Here's how the part is built. I have some questions about the finished solid (model axes, mm). Face numbers are marked on the shaded views. A direction names the side the tool comes from. Coordinates: 2 decimals unless noted, no trailing zeros. Order: outer loops, then holes, each group sorted by start corner. A loop starts at its lowest first (then second) coordinate and runs counter-clockwise, first axis right, second up. Notation, with made-up numbers: (-3, -23.75) - (3, -23.75) arc R27 cw to (3, 14.25) - close; hole circle Ø5 at (45, 4.25). An arc over 180 degrees is marked (long way). Answer as CSV lines item,"result". Start each with the question number.
Q1. For pin 1 Ø0.8 at (x, y) = (-6.5, -16) entering from +Z; pin 2 Ø1.5 at (x, y) = (4.5, -14.5) entering from +Z; pin 3 Ø5 at (x, y) = (0.5, 8) entering from -Z, each with a flat end and sliding along its axis, tell me the tip position at first contact or that it passes through.
Q2. Suppose I cut it at B-B (y = 14). Please give me the cut outline in (x, z), then the cut area to 3 significant figures.
Q3. Suppose I cut it at A-A (x = -6). Please give me the cut outline in (y, z), then the cut area to 3 significant figures.
Q4. For the marked faces 1, 2, 3, 4 and 5, which set-ups out of +Z, -Z, +X, -X, +Y, -Y let a thin tool reach every point of the face, with its end or its side?
Q5. Suppose I cut it at C-C (z = 0). Please give me the cut outline in (x, y), then the cut area to 3 significant figures.
Q6. I need wall thicknesses on line 1 (Y direction, x = -3.25, z = 10); line 2 (Y direction, x = -5.25, z = 3); line 3 (Z direction, x = -3.5, y = 11). Which ranges of each line are inside material? Lowest first, please.
Q7. Suppose I cut it at D-D (z = 9.5). Please give me the cut outline in (x, y), then the cut area to 3 significant figures.
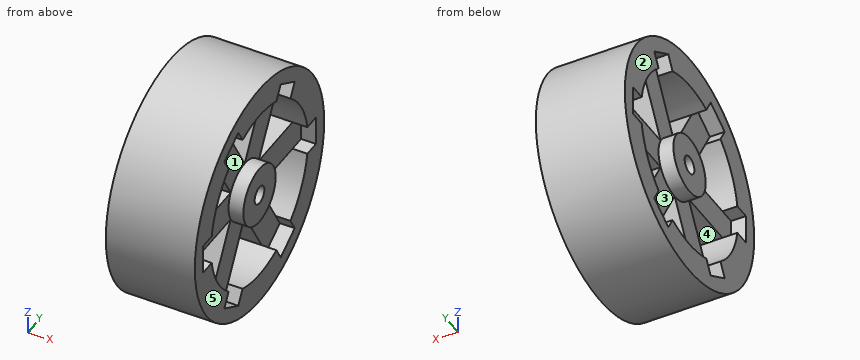
Autodesk Inventor part; units mm, degrees
ref_plane "YZ Plane" through (0, 0, 0) normal (1, 0, 0) x (0, 1, 0)
ref_plane "XZ Plane" through (0, 0, 0) normal (0, 1, 0) x (-1, 0, 0)
ref_plane "XY Plane" through (0, 0, 0) normal (0, 0, 1) x (1, 0, 0)
sketch "Sketch1" plane through (0, 0, 0) normal (1, 0, 0) x (0, 1, 0)
  circle A0 centre (0, 0) radius 20
  circle A1 centre (0, 0) radius 15
  circle A2 centre (0, 0) radius 5
  line L0 (20, 0) -> (9.9317, 0) construction
  line L1 (9.9317, 0) -> (0, 0) construction
  line L2 (17.4317, -2.5) -> (2.4317, -2.5)
  line L3 (2.4317, -2.5) -> (2.4317, 2.5)
  line L4 (2.4317, 2.5) -> (17.4317, 2.5)
  line L5 (17.4317, 2.5) -> (17.4317, -2.5)
  line L6 (17.4317, -2.5) -> (2.4317, 2.5) construction
  line L7 (2.4317, -2.5) -> (17.4317, 2.5) construction
  line L8 (-0.9492, 3.3559) -> (6.5508, 16.3463)
  line L9 (10.8809, 13.8463) -> (3.3809, 0.8559)
  line L10 (6.5508, 16.3463) -> (10.8809, 13.8463)
  line L11 (3.3809, 0.8559) -> (-0.9492, 3.3559)
  line L12 (-3.3809, 0.8559) -> (-10.8809, 13.8463)
  line L13 (-6.5508, 16.3463) -> (0.9492, 3.3559)
  line L14 (-10.8809, 13.8463) -> (-6.5508, 16.3463)
  line L15 (0.9492, 3.3559) -> (-3.3809, 0.8559)
  line L16 (-2.4317, -2.5) -> (-17.4317, -2.5)
  line L17 (-17.4317, 2.5) -> (-2.4317, 2.5)
  line L18 (-17.4317, -2.5) -> (-17.4317, 2.5)
  line L19 (-2.4317, 2.5) -> (-2.4317, -2.5)
  line L20 (0.9492, -3.3559) -> (-6.5508, -16.3463)
  line L21 (-10.8809, -13.8463) -> (-3.3809, -0.8559)
  line L22 (-6.5508, -16.3463) -> (-10.8809, -13.8463)
  line L23 (-3.3809, -0.8559) -> (0.9492, -3.3559)
  line L24 (3.3809, -0.8559) -> (10.8809, -13.8463)
  line L25 (6.5508, -16.3463) -> (-0.9492, -3.3559)
  line L26 (10.8809, -13.8463) -> (6.5508, -16.3463)
  line L27 (-0.9492, -3.3559) -> (3.3809, -0.8559)
  dimension "d0" = 40
  dimension "d1" = 30
  dimension "d2" = 10
  dimension "d4" = 15
  dimension "d5" = 5
  dimension "d8" = 360
extrude "Extrusion1" add sketch "Sketch1" along normal mid plane 15 contours A0 | L4 L3 L11 L15 L13 A2 | L9 L11 L3 L4 | A2 L24 L27 L3 L11 L9 | A2 L20 L23 L27 L3 L2 | L2 L3 L27 L24 | L8 L11 L15 L19 L17 A2 | L13 L15 L11 L8 | L25 L27 L23 L20 | A2 L16 L19 L23 L27 L25 | L12 L15 L19 L23 L21 A2 | L17 L19 L15 L12 | L3 L27 L23 L19 L15 L11 | L21 L23 L19 L16
extrude "Extrusion2" add sketch "Sketch1" along normal mid plane 10 contours A1 L2 A2 L4 | A1 L4 L5 L2 | L9 A2 L8 A1 | A1 L8 L10 L9 | L4 L3 L11 L15 L13 A2 | L9 L11 L3 L4 | A2 L24 L27 L3 L11 L9 | L24 L26 L25 A1 | A1 L25 A2 L24 | A2 L20 L23 L27 L3 L2 | L2 L3 L27 L24 | L8 L11 L15 L19 L17 A2 | L13 L15 L11 L8 | A2 L12 A1 L13 | L20 A1 L21 A2 | L25 L27 L23 L20 | A2 L16 L19 L23 L27 L25 | A1 L12 L14 L13 | L12 L15 L19 L23 L21 A2 | L17 L19 L15 L12 | A2 L16 A1 L17 | L20 L22 L21 A1 | L21 L23 L19 L16 | A1 L16 L18 L17
sketch "Sketch2" plane through (-7.5, 0, 0) normal (-1, 0, 0) x (0, 0, 1)
  circle A0 centre (0, 0) radius 1.5
  dimension "d14" = 3
extrude "Extrusion3" cut sketch "Sketch2" against normal up to next
properties material "Rubber"
Here are the results:
1,pin 1,"stops at z = 12.52"
1,pin 2,"stops at z = 14.52"
1,pin 3,"stops at z = -19.23"
2,outline,"(-7.5, -14.28) - (7.5, -14.28) - (7.5, -5.39) - (-7.5, -5.39) - close; (-7.5, 5.39) - (7.5, 5.39) - (7.5, 14.28) - (-7.5, 14.28) - close; (-5, -2.5) - (5, -2.5) - (5, 2.5) - (-5, 2.5) - close"
2,area,"317 mm²"
3,outline,"circle Ø40 at (0, 0); circle Ø10 at (0, 0); hole (-17.43, -2.5) - (-14.79, -2.5) arc R15 ccw to (-9.56, -11.56) - (-10.88, -13.85) - (-6.55, -16.35) - (-5.23, -14.06) arc R15 ccw to (5.23, -14.06) - (6.55, -16.35) - (10.88, -13.85) - (9.56, -11.56) arc R15 ccw to (14.79, -2.5) - (17.43, -2.5) - (17.43, 2.5) - (14.79, 2.5) arc R15 ccw to (9.56, 11.56) - (10.88, 13.85) - (6.55, 16.35) - (5.23, 14.06) arc R15 ccw to (-5.23, 14.06) - (-6.55, 16.35) - (-10.88, 13.85) - (-9.56, 11.56) arc R15 ccw to (-14.79, 2.5) - (-17.43, 2.5) - close; hole circle Ø3 at (0, 0)"
3,area,"546 mm²"
4,face 1,"+X"
4,face 2,"+Z, -Z, -X, +Y, -Y"
4,face 3,"-X"
4,face 4,"+X, -X"
4,face 5,"+Z, -Z, +X, +Y, -Y"
5,outline,"(-7.5, -20) - (7.5, -20) - (7.5, -17.43) - (5, -17.43) - (5, -5) - (7.5, -5) - (7.5, -1.5) - (-7.5, -1.5) - (-7.5, -5) - (-5, -5) - (-5, -17.43) - (-7.5, -17.43) - close; (-7.5, 1.5) - (7.5, 1.5) - (7.5, 5) - (5, 5) - (5, 17.43) - (7.5, 17.43) - (7.5, 20) - (-7.5, 20) - (-7.5, 17.43) - (-5, 17.43) - (-5, 5) - (-7.5, 5) - close"
5,area,"431 mm²"
6,line 1,"y = -17.32 to -11.18, -8.66 to -2.89, 2.89 to 8.66, 11.18 to 17.32"
6,line 2,"y = -19.77 to -14.7, -4 to 4, 14.7 to 19.77"
6,line 3,"z = -16.7 to -10.2, -2.5 to 2.5, 10.2 to 16.7"
7,outline,"(-7.5, -17.6) - (7.5, -17.6) - (7.5, -11.61) - (-7.5, -11.61) - close; (-7.5, 11.61) - (7.5, 11.61) - (7.5, 17.6) - (-7.5, 17.6) - close; (-5, -8.37) - (5, -8.37) - (5, -2.6) - (-5, -2.6) - close; (-5, 2.6) - (5, 2.6) - (5, 8.37) - (-5, 8.37) - close"
7,area,"295 mm²"
